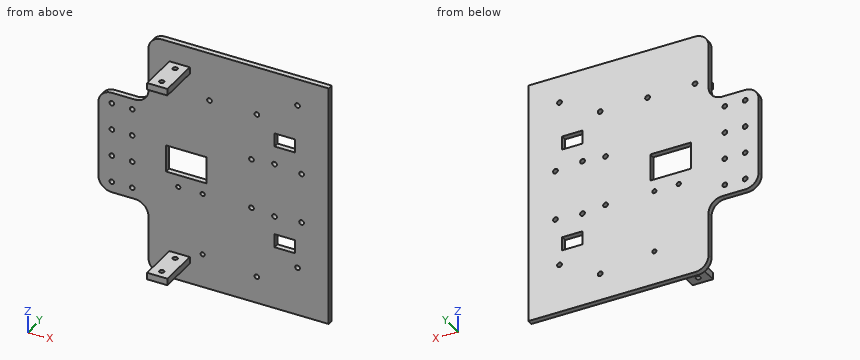
from build123d import *

# Parameters (mm, degrees)
SKETCH1_W               = 300
SKETCH1_H               = 180
MAIN_BODY_DEPTH         = 4
FILLET1_R               = 10
CHAMFER1_SIZE           = 10
SKETCH2_R               = 1.75
BATTERIES_HOLES_DEPTH   = 15
SKETCH5_R               = 1.75
SKETCH5_W               = 15
SKETCH5_H               = 10
L298N_HOLES_DEPTH       = 15
SKETCH6_R               = 1.75
LM2596_HOLES_DEPTH      = 15
SKETCH7_R               = 1.55
ESP32_HOLES_DEPTH       = 15
SKETCH8_R               = 1.75
PCB_SENSORS_HOLES_DEPTH = 15
SKETCH9_W               = 15
SKETCH9_H               = 5
WHEELS_LEGS_DEPTH       = 30
SKETCH10_R              = 1.75
MOTOR_HOLES_DEPTH       = 300
SKETCH11_R              = 1.75
SKETCH11_W              = 30
SKETCH11_H              = 20
SENSORS_HOLES_DEPTH     = 15
SKETCH13_W              = 40
SKETCH13_H              = 75
CUT_EXTRUDE2_DEPTH      = 10
FILLET2_R               = 10
SKETCH12_R              = 1.75
CUT_EXTRUDE3_DEPTH      = 10
SKETCH14_W              = 219.25277831
SKETCH14_H              = 99.771872263
CUT_EXTRUDE4_DEPTH      = 200


with BuildPart() as part:
    # Sketch1 → Main Body (new body)
    with BuildSketch(Plane(origin=(0, 0, 0), x_dir=(1, 0, 0), z_dir=(0, 1, 0))):
        Rectangle(SKETCH1_W, SKETCH1_H)
    extrude(amount=MAIN_BODY_DEPTH)

    # Fillet1
    fillet1_edges = [part.edges().sort_by_distance(p)[0] for p in [
        (-150, 2, 90),
        (-150, 2, -90),
    ]]
    fillet(fillet1_edges, radius=FILLET1_R)

    # Chamfer1
    chamfer1_edges = [part.edges().sort_by_distance(p)[0] for p in [
        (150, 2, 90),
        (150, 2, -90),
    ]]
    chamfer(chamfer1_edges, length=CHAMFER1_SIZE)

    # Sketch2 → Batteries holes (cut)
    with BuildSketch(Plane(origin=(0, 4, 0), x_dir=(1, 0, 0), z_dir=(0, 1, 0))):
        with Locations(Location((115, 75, 0), (0, 0, 270))):
            Circle(SKETCH2_R)
        with Locations(Location((115, 14, 0), (0, 0, 270))):
            Circle(SKETCH2_R)
        with Locations(Location((115, -14, 0), (0, 0, 90))):
            Circle(SKETCH2_R)
        with Locations(Location((115, -75, 0), (0, 0, 90))):
            Circle(SKETCH2_R)
        with Locations(Location((45, -75, 0), (0, 0, 270))):
            Circle(SKETCH2_R)
        with Locations(Location((45, -14, 0), (0, 0, 270))):
            Circle(SKETCH2_R)
        with Locations(Location((45, 14, 0), (0, 0, 90))):
            Circle(SKETCH2_R)
        with Locations(Location((45, 75, 0), (0, 0, 90))):
            Circle(SKETCH2_R)
    extrude(amount=-BATTERIES_HOLES_DEPTH, mode=Mode.SUBTRACT)

    # Sketch5 → L298N holes (cut)
    with BuildSketch(Plane(origin=(0, 4, 0), x_dir=(1, 0, 0), z_dir=(0, 1, 0))):
        with Locations(Location((-37, 18.5, 0), (0, 0, 270))):
            Circle(SKETCH5_R)
        with Locations(Location((0, 18.5, 0), (0, 0, 270))):
            Circle(SKETCH5_R)
        with Locations(Location((-37, -18.5, 0), (0, 0, 270))):
            Circle(SKETCH5_R)
        with Locations(Location((0, -18.5, 0), (0, 0, 270))):
            Circle(SKETCH5_R)
        with Locations((-12.5, -38.5)):
            Rectangle(SKETCH5_W, SKETCH5_H)
        with Locations((-12.5, 38.5)):
            Rectangle(SKETCH5_W, SKETCH5_H)
    extrude(amount=-L298N_HOLES_DEPTH, mode=Mode.SUBTRACT)

    # Sketch6 → LM2596 holes (cut)
    with BuildSketch(Plane(origin=(0, 4, 0), x_dir=(1, 0, 0), z_dir=(0, 1, 0))):
        with Locations(Location((-33, 70, 0), (0, 0, 270))):
            Circle(SKETCH6_R)
        with Locations(Location((-3, 54, 0), (0, 0, 270))):
            Circle(SKETCH6_R)
        with Locations(Location((-33, -54, 0), (0, 0, 270))):
            Circle(SKETCH6_R)
        with Locations(Location((-3, -70, 0), (0, 0, 270))):
            Circle(SKETCH6_R)
    extrude(amount=-LM2596_HOLES_DEPTH, mode=Mode.SUBTRACT)

    # Sketch7 → ESP32 holes (cut)
    with BuildSketch(Plane(origin=(0, 4, 0), x_dir=(1, 0, 0), z_dir=(0, 1, 0))):
        with Locations(Location((-73, 65, 0), (0, 0, 270))):
            Circle(SKETCH7_R)
        with Locations(Location((-73, 19, 0), (0, 0, 270))):
            Circle(SKETCH7_R)
        with Locations(Location((-91, 19, 0), (0, 0, 270))):
            Circle(SKETCH7_R)
    extrude(amount=-ESP32_HOLES_DEPTH, mode=Mode.SUBTRACT)

    # Sketch8 → PCB sensors holes (cut)
    with BuildSketch(Plane(origin=(0, 4, 0), x_dir=(1, 0, 0), z_dir=(0, 1, 0))):
        with Locations(Location((-103, -54, 0), (0, 0, 270))):
            Circle(SKETCH8_R)
        with Locations(Location((-68, -54, 0), (0, 0, 90))):
            Circle(SKETCH8_R)
    extrude(amount=-PCB_SENSORS_HOLES_DEPTH, mode=Mode.SUBTRACT)

    # Sketch9 → Wheels legs (add)
    with BuildSketch(Plane.XZ):
        with Locations((-90, 72.5)):
            Rectangle(SKETCH9_W, SKETCH9_H)
        with Locations((90, 72.5)):
            Rectangle(SKETCH9_W, SKETCH9_H)
        with Locations((90, -72.5)):
            Rectangle(SKETCH9_W, SKETCH9_H)
        with Locations((-90, -72.5)):
            Rectangle(SKETCH9_W, SKETCH9_H)
    extrude(amount=WHEELS_LEGS_DEPTH)

    # Sketch10 → Motor holes (cut)
    with BuildSketch(Plane.XY.offset(75)):
        with Locations((-90, -24)):
            Circle(SKETCH10_R)
        with Locations((-90, -6)):
            Circle(SKETCH10_R)
        with Locations((90, -6)):
            Circle(SKETCH10_R)
        with Locations((90, -24)):
            Circle(SKETCH10_R)
    extrude(amount=-MOTOR_HOLES_DEPTH, mode=Mode.SUBTRACT)

    # Sketch11 → Sensors holes (cut)
    with BuildSketch(Plane(origin=(0, 4, 0), x_dir=(1, 0, 0), z_dir=(0, 1, 0))):
        with Locations(Location((-140, 10, 0), (0, 0, 270))):
            Circle(SKETCH11_R)
        with Locations(Location((-125, 10, 0), (0, 0, 270))):
            Circle(SKETCH11_R)
        with Locations(Location((-125, 30, 0), (0, 0, 90))):
            Circle(SKETCH11_R)
        with Locations(Location((-140, 30, 0), (0, 0, 90))):
            Circle(SKETCH11_R)
        with Locations(Location((-125, -30, 0), (0, 0, 270))):
            Circle(SKETCH11_R)
        with Locations(Location((-140, -30, 0), (0, 0, 270))):
            Circle(SKETCH11_R)
        with Locations(Location((-125, -10, 0), (0, 0, 90))):
            Circle(SKETCH11_R)
        with Locations(Location((-140, -10, 0), (0, 0, 90))):
            Circle(SKETCH11_R)
        with Locations((-85, 0)):
            Rectangle(SKETCH11_W, SKETCH11_H)
    extrude(amount=-SENSORS_HOLES_DEPTH, mode=Mode.SUBTRACT)

    # Sketch13 → Cut-Extrude2 (cut)
    with BuildSketch(Plane.XZ):
        with Locations((-133, 75.5)):
            Rectangle(SKETCH13_W, SKETCH13_H)
        with Locations((-133, -75.5)):
            Rectangle(SKETCH13_W, SKETCH13_H)
    extrude(amount=-CUT_EXTRUDE2_DEPTH, mode=Mode.SUBTRACT)

    # Fillet2
    fillet2_edges = [part.edges().sort_by_distance(p)[0] for p in [
        (-113, 2, 90),
        (-150, 2, 38),
        (-113, 2, 38),
        (-113, 2, -90),
        (-113, 2, -38),
        (-150, 2, -38),
    ]]
    fillet(fillet2_edges, radius=FILLET2_R)

    # Sketch12 → Cut-Extrude3 (cut)
    with BuildSketch(Plane(origin=(0, 4, 0), x_dir=(1, 0, 0), z_dir=(0, 1, 0))):
        with Locations(Location((80, 20, 0), (0, 0, 270))):
            Circle(SKETCH12_R)
        with Locations(Location((80, -20, 0), (0, 0, 90))):
            Circle(SKETCH12_R)
        with Locations(Location((-20, -20, 0), (0, 0, 270))):
            Circle(SKETCH12_R)
        with Locations(Location((-20, 20, 0), (0, 0, 90))):
            Circle(SKETCH12_R)
    extrude(amount=-CUT_EXTRUDE3_DEPTH, mode=Mode.SUBTRACT)

    # Sketch14 → Cut-Extrude4 (cut)
    with BuildSketch(Plane.ZY.offset(-20)):
        with Locations((0.286230781, -6.766483263)):
            Rectangle(SKETCH14_W, SKETCH14_H)
    extrude(amount=-CUT_EXTRUDE4_DEPTH, mode=Mode.SUBTRACT)


solid = part.part
Design review of the part built by this model. Coordinates are the model's own, in mm. Round coordinates to 2 decimals unless told otherwise and drop trailing zeros. Write each loop counter-clockwise with the first axis right and the second up, starting at its lowest first coordinate (ties: lowest second). Pieces come first, ordered by that corner, then holes. Notation, with made-up numbers: (26.5, 80.5) - (70.5, 80.5) arc R19 cw to (70.5, 110.5) - close; hole circle Ø10 at (-21.5, 46). An arc over 180 degrees is marked (long way). Return JSON: item names as keys, results as strings. Group by question number.
Item 1: For probe 1 along Z at (x, y) = (-73, 0.95); probe 2 along X at (y, z) = (0.8, -65); probe 3 along X at (y, z) = (2.8, 54), list the stretches that pass through material, from the lowest coordinate up. Write a range as [from, to].
Item 2: We need section B-B on x = -134. Write out the cut boundary in (y, z).
Item 3: We need section A-A on y = -19.5. Write out the cut boundary in (x, z), and give its area (3 significant figures).
Item 4: Insertion check: P1, Ø1.5, axis at x = -92.5, y = -2.5, coming from the -Z side; P2, Ø3, axis at x = -37, z = -18.5, coming from the +Y side; P3, Ø10, axis at x = -1.5, z = -39.5, coming from the -Y side; P4, Ø3, axis at x = -132, y = 1.5, coming from the -Z side. Each pin has a flat end and moves straight along its axis. Give the tip position at first contact, or say it passes through.
Model answer:
{
 "1": {"probe 1": "z = [-90, -66.55], [-63.45, -20.55], [-17.45, -10], [10, 90]", "probe 2": "x = [-113, -74.55], [-71.45, 20]", "probe 3": "x = [-113, -104.75], [-101.25, -69.75], [-66.25, -34.75], [-31.25, 20]"},
 "2": {"outline": "(0, -38) - (4, -38) - (4, 38) - (0, 38) - close"},
 "3": {"outline": "(-97.5, -75) - (-82.5, -75) - (-82.5, -70) - (-97.5, -70) - close; (-97.5, 70) - (-82.5, 70) - (-82.5, 75) - (-97.5, 75) - close", "area": "150 mm²"},
 "4": {"P1": "stops at z = -75", "P2": "passes through", "P3": "stops at y = 0", "P4": "stops at z = -38"}
}
